```python
from build123d import *

# Parameters (mm, degrees)
BOSS_EXTRUDE5_DEPTH = 234.9999999
SKETCH4_W           = 42.5
SKETCH4_H           = 48.09999997
CUT_EXTRUDE1_DEPTH  = 2.000000064
RIB1_REACH          = 504.592
SKETCH9_WALLS_W     = 1213.053497679
SKETCH9_WALLS_H     = 2.54
RIB2_REACH          = 504.592
SKETCH8_WALLS_W     = 1213.053497679
SKETCH8_WALLS_H     = 2.54


with BuildPart() as part:
    # Sketch1 → Boss-Extrude5 (new body)
    with BuildSketch(Plane(origin=(0, 0, 0), x_dir=(1, 0, 0), z_dir=(0, 1, 0))):
        Polygon((-117.504462868, 326.155640462), (117.504462868, 326.155640462), (263.000000064, 160.754471715), (263.000000064, 45.003453118), (261, 45.003453118), (261, 160), (116.600094822, 324.155640398), (-116.600094822, 324.155640398), (-261, 160), (-261, 45.001214275), (-263.000000064, 45.001214275), (-263.000000064, 160.754471715), align=None)
    extrude(amount=BOSS_EXTRUDE5_DEPTH)

    # Sketch4 → Cut-Extrude1 (cut)
    with BuildSketch(Plane(origin=(0, 0, -326.155640462), x_dir=(-1, 0, 0), z_dir=(0, 0, -1))):
        with Locations((0, 87.449999931)):
            Rectangle(SKETCH4_W, SKETCH4_H)
        Polygon((-25, 63.399999946), (-25, 28.4), (25, 28.4), (25, 63.399999946), (21.25, 63.399999946), (-21.25, 63.399999946), align=None)
        Polygon((-25, 28.4), (-35, 28.4), (-35, 0), (35, 0), (35, 28.4), (25, 28.4), align=None)
    extrude(amount=-CUT_EXTRUDE1_DEPTH, mode=Mode.SUBTRACT)

    # Sketch9 walls → Rib1 (add, up to next)
    with BuildSketch(Plane(origin=(118.5216607, 0, -272.630231957), x_dir=(0.917086319794662, 0, 0.39868870318267463), z_dir=(-0.39868870318267463, 0, 0.917086319794662)), mode=Mode.PRIVATE) as rib1_sk1:
        with Locations((-26.302471723, 220.03320014)):
            Rectangle(SKETCH9_WALLS_W, SKETCH9_WALLS_H)
    rib1_tool1 = extrude(rib1_sk1.sketch, amount=-RIB1_REACH, mode=Mode.PRIVATE) - part.part
    add(rib1_tool1.solids().sort_by_distance((94.400023705, 220.03320014, -283.116730299))[0])

    # Sketch8 walls → Rib2 (add, up to next)
    with BuildSketch(Plane(origin=(-118.5216607, 0, -272.630231957), x_dir=(0.9170863197945202, 0, -0.39868870318300126), z_dir=(0.3986887031830012, 0, 0.91708631979452)), mode=Mode.PRIVATE) as rib2_sk1:
        with Locations((26.302471723, 220.03320014)):
            Rectangle(SKETCH8_WALLS_W, SKETCH8_WALLS_H)
    rib2_tool1 = extrude(rib2_sk1.sketch, amount=-RIB2_REACH, mode=Mode.PRIVATE) - part.part
    add(rib2_tool1.solids().sort_by_distance((-94.400023705, 220.03320014, -283.116730299))[0])


solid = part.part
```
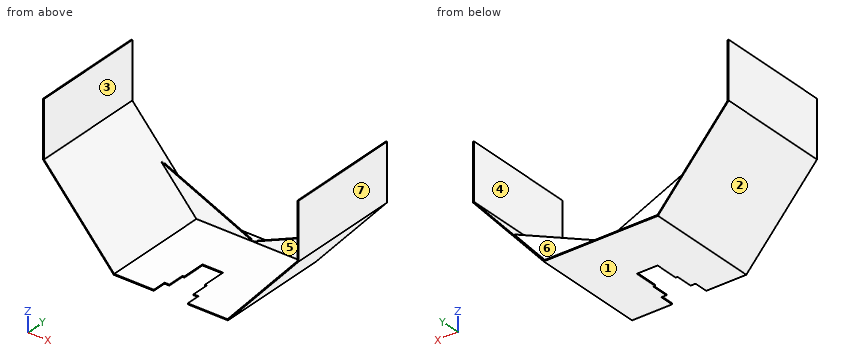
Geometry: final body of the model. Coordinates: model frame, mm. Face numbers are marked on the shaded views. A direction names the side the tool comes from. Round coordinates to 2 decimals unless told otherwise and drop trailing zeros. Write each loop counter-clockwise with the first axis right and the second up, starting at its lowest first coordinate (ties: lowest second). Pieces come first, ordered by that corner, then holes. Notation, with made-up numbers: (35, 12) -> (51, 12) arc R30 cw to (51, 51) -> close; hole circle Ø1 at (-1, -10). An arc over 180 degrees is marked (long way). Use CSV: the item, a comma, the result in double quotes. Start each with the question number.
Q1. Pull-direction query (X, two-part tool) for the marked faces 1, 2 and 3; classes: pulls with the +X half, pulls with the -X half, needs draft (parallel to the pull), parting line crosses it, or undercut.
Q2. Section D-D (x = 107). Return loops of the section in (y, z), plus the area to 3 significant figures.
Q3. Section A-A (y = 87.5). Return loops of the section in (x, z), plus the area to 3 significant figures.
Q4. Section B-B (z = -115). Return loops of the section in (x, y).
Q5. Section C-C (y = 36). Return loops of the section in (x, z).
Q6. First-contact query: pin 1 Ø2 at (y, z) = (12.5, -325) entering from -X; pin 2 Ø8 at (y, z) = (134, -278) entering from -X; pin 3 Ø12 at (x, y) = (168, 82.5) entering from -Z. Flat tips, straight axial feed; report the tip coordinate or a pass-through.
Q7. Line query: L1, parallel to X at y = 59, z = -61; L2, parallel to X at y = 183, z = -195; L3, parallel to Z at x = -63, y = 133.5. Output: solid intervals per line, ascending.
Q8. Reachability of the marked faces 4, 5, 6 and 7 from +Z, -Z, +X, -X, +Y, -Y: full face, straight path, thin tool, end or side. Return the list, or none.
Result sheet:
1,face 1,"needs draft"
1,face 2,"pulls with the -X half"
1,face 3,"undercut"
2,outline,"(0, -326.16) -> (235, -326.16) -> (235, -324.16) -> (221.3, -324.16) -> (221.3, -277.64) -> (218.76, -277.64) -> (218.76, -324.16) -> (0, -324.16) -> close"
2,area,"588 mm²"
3,outline,"(-263, -160.75) -> (-117.5, -326.16) -> (-21.25, -326.16) -> (-21.25, -324.16) -> (-116.6, -324.16) -> (-261, -160) -> (-261, -45) -> (-263, -45) -> close; (21.25, -326.16) -> (117.5, -326.16) -> (263, -160.75) -> (263, -45) -> (261, -45) -> (261, -160) -> (116.6, -324.16) -> (21.25, -324.16) -> close"
3,area,"1,720 mm²"
4,outline,"(-263, 0) -> (-261, 0) -> (-261, 235) -> (-263, 235) -> close; (261, 0) -> (263, 0) -> (263, 235) -> (261, 235) -> close"
5,outline,"(-263, -160.75) -> (-117.5, -326.16) -> (-25, -326.16) -> (-25, -324.16) -> (-116.6, -324.16) -> (-261, -160) -> (-261, -45) -> (-263, -45) -> close; (25, -326.16) -> (117.5, -326.16) -> (263, -160.75) -> (263, -45) -> (261, -45) -> (261, -160) -> (116.6, -324.16) -> (25, -324.16) -> close"
6,pin 1,"x = -119.4"
6,pin 2,"x = -163.38"
6,pin 3,"z = -275.57"
7,L1,"-263 to -261, 261 to 263"
7,L2,"-232.88 to -230.21, 230.21 to 232.88"
7,L3,"-326.16 to -324.16"
8,face 4,"+Z, +Y, -Y"
8,face 5,"+Z, -Y"
8,face 6,"+Z, +Y"
8,face 7,"+Z, -Z, +X, +Y, -Y"
